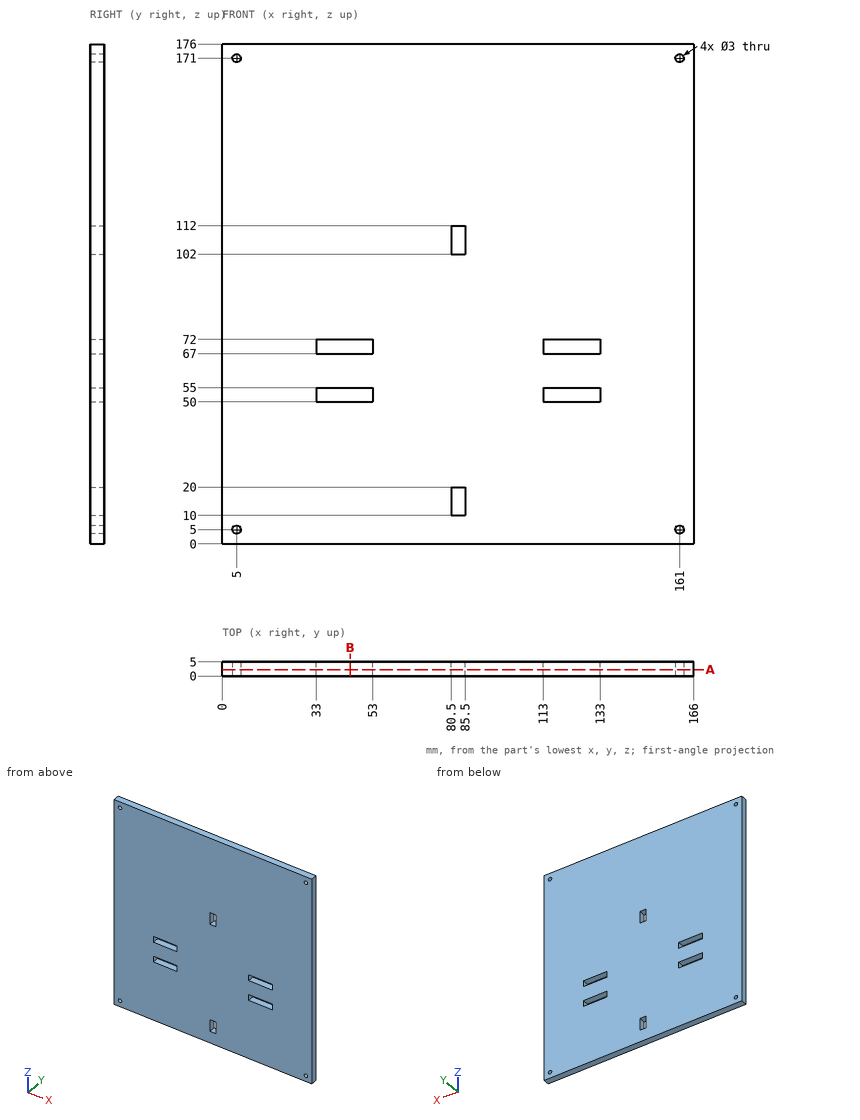
Part print with two shaded views. Sizes in mm from the minimum x, y, z corner. Coordinates: 2 decimals unless noted, no trailing zeros. Loops run counter-clockwise (first coordinate to the right, second up) from the corner with the lowest first, then second, coordinate; pieces in that order, holes last. Notation, with made-up numbers: (6.25, 38) - (56.25, 38) arc R28 cw to (56.25, 75) - close; hole circle Ø1 at (89, -0.75). An arc over 180 degrees is marked (long way). Write each question's results on one line, items separated by ' | '. Start each with the question number.
Q1. Slice it at B-B on x = 45. Give the cut face in (y, z).
Q2. Probe line 1 along X through (y, z) = (3.4, 5); line 2 along Z through (x, y) = (127.5, 2.65); line 3 along Z through (x, y) = (161, 2.35). List the from-to ranges inside material, lowest first.
Q3. Slice it at A-A on y = 2.25. Give the number of separate pieces and of enclosed holes in the cut face, and give its area (3 significant figures).
Answer:
1) outline: (0, 0) - (5, 0) - (5, 50) - (0, 50) - close; (0, 55) - (5, 55) - (5, 67) - (0, 67) - close; (0, 72) - (5, 72) - (5, 176) - (0, 176) - close
2) line 1: x = 0 to 3.5, 6.5 to 159.5, 162.5 to 166 | line 2: z = 0 to 50, 55 to 67, 72 to 176 | line 3: z = 0 to 3.5, 6.5 to 169.5, 172.5 to 176
3) separate pieces: 1 | enclosed holes: 10 | area: 28,700 mm2
